CAD build for the part. Positions are in the model's coordinates, mm. A direction names the side the tool comes from. Give positions to 0.01 mm unless a question says otherwise; leave off trailing zeros. Write each loop counter-clockwise with the first axis right and the second up, starting at its lowest first coordinate (ties: lowest second). Pieces come first, ordered by that corner, then holes. Notation, with made-up numbers: (62.25, 83.25) -> (83.25, 83.25) arc R26 cw to (83.25, 115.25) -> close; hole circle Ø5 at (-0.75, 26). An arc over 180 degrees is marked (long way). Answer as a JSON object with one key per item and string values.
Autodesk Inventor part; units mm, degrees
ref_plane "YZ Plane" through (0, 0, 0) normal (1, 0, 0) x (0, 1, 0)
ref_plane "XZ Plane" through (0, 0, 0) normal (0, 1, 0) x (-1, 0, 0)
ref_plane "XY Plane" through (0, 0, 0) normal (0, 0, 1) x (1, 0, 0)
sketch "Sketch1" plane through (0, 0, 0) normal (0, 1, 0) x (-1, 0, 0)
  line L0 (0, 0) -> (30, 0)
  line L1 (30, 0) -> (30, -110)
  line L2 (30, -110) -> (0, -110)
  line L3 (0, -110) -> (0, 0)
  line L4 (6.5, -110) -> (23.5, -110)
  line L5 (23.5, -110) -> (23.5, -70)
  line L6 (23.5, -70) -> (6.5, -70)
  line L7 (6.5, -70) -> (6.5, -110)
  circle A0 centre (26.5, -103) radius 1
  circle A1 centre (3.5, -103) radius 1
  line L8 (30, -105) -> (0, -105) construction
  circle A2 centre (26.5, -90.5) radius 1
  circle A3 centre (3.5, -90.5) radius 1
  line L9 (22.4, 0) -> (7.6, 0)
  line L10 (7.6, 0) -> (7.6, -55)
  line L11 (7.6, -55) -> (22.4, -55)
  line L12 (22.4, -55) -> (22.4, 0)
  line L13 (22.4, -55) -> (30, -62.6)
  line L14 (22.4, -55) -> (33.148, -55) construction
  line L15 (7.6, -55) -> (0, -62.6)
  line L16 (7.6, -55) -> (18.348, -55) construction
  point P0 (27.5, -90.5)
  point P1 (2.5, -90.5)
  point P2 (15, 0)
  point P3 (15, -55)
  point P4 (15, -70)
  point P5 (22.4, 0)
  point P6 (7.6, 0)
  dimension "d0" = 30
  dimension "d1" = 110
  dimension "d2" = 2
  dimension "d3" = 2
  dimension "d4" = 14.5
  dimension "d5" = 5
  dimension "d6" = 25
  dimension "d7" = 3
  dimension "d8" = 3
  dimension "d11" = 3.5
  dimension "d12" = 3.5
  dimension "d13" = 40
  dimension "d19" = 14.8
  dimension "d20" = 55
  dimension "d21" = 45
  dimension "d22" = 135
extrude "Extrusion1" add sketch "Sketch1" along normal blind 4.8 contours L0 L12 L11 L10 | L15 L11 L13 L1 L2 L5 L6 L7 L3
chamfer "Chamfer1" distance 3 angle 45 4 edges at (-23.5, 2.4, -70) (-6.5, 2.4, -70) (-30, 2.4, -110) (0, 2.4, -110)
properties part number "camera_holder"
1) Pin check, flat tips, straight feed: pin 1 (1.2 mm diameter, centred on x = -3.5, z = -103, fed in from -Y); pin 2 (1 mm diameter, centred on x = -22.5, y = 3, fed in from -Z); pin 3 (2 mm diameter, centred on x = -16.5, y = 1, fed in from -Z); pin 4 (1.4 mm diameter, centred on y = 1.5, z = -36, fed in from +X). Stop position of each tip, or through.
Model answer:
{"pin 1": "passes through", "pin 2": "stops at z = -72.5", "pin 3": "stops at z = -70", "pin 4": "stops at x = -7.6"}
2) Slice it at D-D (z = -49). List the corners of the cut face in (x, y), then the cut area to 3 significant figures.
Model answer:
{"outline": "(-22.4, 0) -> (-7.6, 0) -> (-7.6, 4.8) -> (-22.4, 4.8) -> close", "area": "71.0 mm2"}
3) Wall check: probe 1 along X at (y, z) = (1.75, -103); probe 2 along X at (y, z) = (3.7, -85.5); probe 3 along Z at (x, y) = (-26.5, 2.2). Give the ranges that are in metal, low to high.
Model answer:
{"probe 1": "x = -30 to -27.5, -25.5 to -23.5, -6.5 to -4.5, -2.5 to 0", "probe 2": "x = -30 to -23.5, -6.5 to 0", "probe 3": "z = -110 to -104, -102 to -91.5, -89.5 to -59.1"}
4) Slice it at A-A (z = -90.5). List the corners of the cut face in (x, y), then the cut area to 3 significant figures.
Model answer:
{"outline": "(-30, 0) -> (-27.5, 0) -> (-27.5, 4.8) -> (-30, 4.8) -> close; (-25.5, 0) -> (-23.5, 0) -> (-23.5, 4.8) -> (-25.5, 4.8) -> close; (-6.5, 0) -> (-4.5, 0) -> (-4.5, 4.8) -> (-6.5, 4.8) -> close; (-2.5, 0) -> (0, 0) -> (0, 4.8) -> (-2.5, 4.8) -> close", "area": "43.2 mm2"}
5) Slice it at B-B (y = 3.8). List the corners of the cut face in (x, z), then the cut area to 3 significant figures.
Model answer:
{"outline": "(-30, -107) -> (-27, -110) -> (-23.5, -110) -> (-23.5, -73) -> (-20.5, -70) -> (-9.5, -70) -> (-6.5, -73) -> (-6.5, -110) -> (-3, -110) -> (0, -107) -> (0, -62.6) -> (-7.6, -55) -> (-7.6, 0) -> (-22.4, 0) -> (-22.4, -55) -> (-30, -62.6) -> close; hole circle Ø2 at (-26.5, -103); hole circle Ø2 at (-26.5, -90.5); hole circle Ø2 at (-3.5, -103); hole circle Ø2 at (-3.5, -90.5)", "area": "1,710 mm2"}
6) 3-axis set-ups, long thin cutter, end or side, ignore diameter. For faces 5 (the flat face through (-8, 2.4, -71.5)), 6 (the flat face through (-30, 2, -84)), 7 (the flat face through (-22.4, 2, -28)): which of +Z, -Z, +X, -X, +Y, -Y reach the whole face in a straight line?
Model answer:
{"face 5": "-Z, +Y, -Y", "face 6": "+Z, -Z, -X, +Y, -Y", "face 7": "+Z, -X, +Y, -Y"}
7) Mould opens along X. For faces 1 (the cylindrical face through (-26.96, 2.37, -89.61)), 2 (the cylindrical face through (-26.96, 2.37, -102.11)), 3 (the flat face through (-7.6, 2, -27)), 4 (the flat face through (-15, 2, 0)) say: released by +X, released by -X, zero draft, split by the parting line, or undercut.
Model answer:
{"face 1": "undercut", "face 2": "undercut", "face 3": "released by +X", "face 4": "zero draft"}
8) Slice it at C-C (x = -13.75). List the corners of the cut face in (y, z).
Model answer:
{"outline": "(0, -70) -> (4.8, -70) -> (4.8, 0) -> (0, 0) -> close"}
